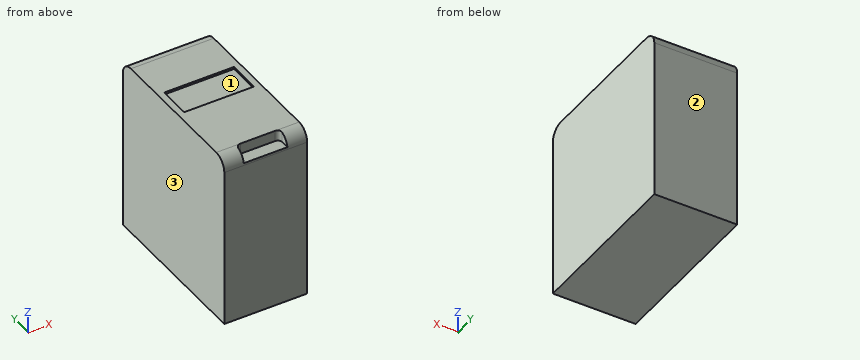
from build123d import *

# Parameters (mm, degrees)
CROQUIS1_W              = 400
CROQUIS1_H              = 380
SALIENTE_EXTRUIR1_DEPTH = 95
REDONDEO1_R             = 30
CROQUIS2_W              = 160
CROQUIS2_H              = 75
CORTAR_EXTRUIR1_DEPTH   = 5
CORTAR_EXTRUIR2_DEPTH   = 25


with BuildPart() as part:
    # Croquis1 → Saliente-Extruir1 (new body, symmetric)
    with BuildSketch(Plane(origin=(0, 0, 0), x_dir=(0, 0, -1), z_dir=(1, 0, 0))):
        Rectangle(CROQUIS1_W, CROQUIS1_H)
    extrude(amount=SALIENTE_EXTRUIR1_DEPTH, both=True)

    # Redondeo1
    redondeo1_edges = [part.edges().sort_by_distance(p)[0] for p in [
        (0, 190, 200),
        (0, -190, 200),
    ]]
    fillet(redondeo1_edges, radius=REDONDEO1_R)

    # Croquis2 → Cortar-Extruir1 (cut)
    with BuildSketch(Plane.XY.offset(200)):
        with Locations((0, 22.171988643)):
            Rectangle(CROQUIS2_W, CROQUIS2_H)
    extrude(amount=-CORTAR_EXTRUIR1_DEPTH, mode=Mode.SUBTRACT)

    # Croquis3 → Cortar-Extruir2 (cut)
    with BuildSketch(Plane.XY.offset(200)):
        with BuildLine():
            Line((40, -160), (-40, -160))
            ThreePointArc((-40, -160), (-47.071067812, -162.928932188), (-50, -170))
            Line((-50, -170), (-50, -190))
            Line((-50, -190), (50, -190))
            Line((50, -190), (50, -170))
            ThreePointArc((50, -170), (47.071067812, -162.928932188), (40, -160))
        make_face()
    extrude(amount=-CORTAR_EXTRUIR2_DEPTH, mode=Mode.SUBTRACT)


solid = part.part
Geometry: final body of the model. Coordinates: model frame, mm. Face numbers are marked on the shaded views. Coordinates: 2 decimals unless noted, no trailing zeros.
(1) Draft query along Y for the marked faces 1, 2 and 3. Return one class per face: pulls with the +Y half, pulls with the -Y half, needs draft (parallel to the pull), parting line crosses it, or undercut.
(2) Material intervals for probe 1 along Z at (x, y) = (-24.5, 32.5); probe 2 along Y at (x, z) = (28.5, 173); probe 3 along Z at (x, y) = (-69.5, -165.5), sorted ascending.
(3) First-contact query: pin 1 (15 mm diameter, centred on x = -3, y = -175.5, fed in from +Z); pin 2 (4 mm diameter, centred on x = 21.5, z = 198, fed in from -Y); pin 3 (3 mm diameter, centred on x = 34, y = -0.5, fed in from +Z). Flat tips, straight axial feed; report the tip coordinate or a pass-through.
Solution:
1. face 1: undercut
1. face 2: pulls with the +Y half
1. face 3: needs draft
2. probe 1: z = -200 to 195
2. probe 2: y = -189.85 to 189.85
2. probe 3: z = -200 to 199.49
3. pin 1: stops at z = 175
3. pin 2: stops at y = -160
3. pin 3: stops at z = 195
